Design review of the part shown in the three views and the two pictorial views. Dimensions are in mm from the part's minimum x, y and z. Give positions to 0.01 mm unless a question says otherwise; leave off trailing zeros. Loops run counter-clockwise (first coordinate to the right, second up) from the corner with the lowest first, then second, coordinate; pieces in that order, holes last. Notation, with made-up numbers: (-27, 12.5) - (17, 12.5) arc R17 ccw to (17, 31.5) - close; hole circle Ø6 at (24, 64). An arc over 180 degrees is marked (long way). Answer in a Markdown table with one row per item.
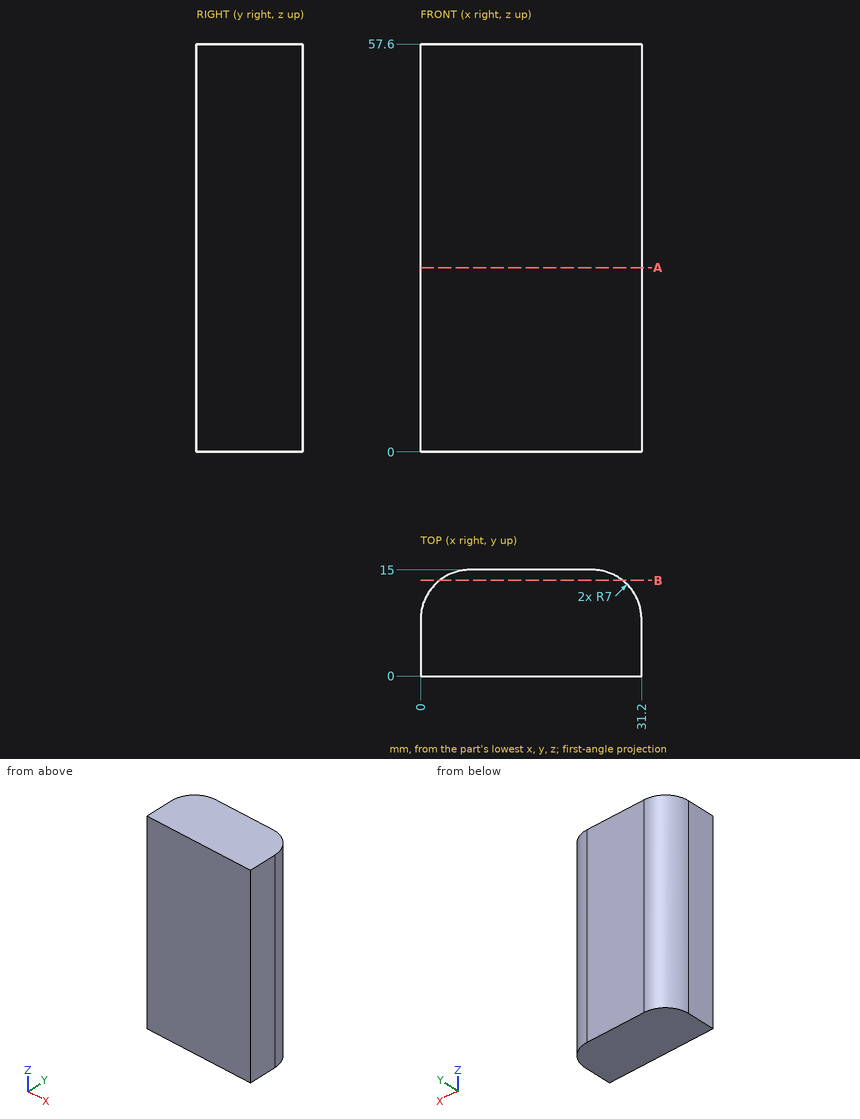
1. Wall thickness on line 1 (Y direction, x = 2, z = 21.5); line 2 (Y direction, x = 27.5, z = 33); line 3 (X direction, y = 11.5, z = 43): over which ranges is each line inside the solid? List them lowest first. Write a range as [from, to].
Values:
| item | result |
|---|---|
| line 1 | y = [0, 12.9] |
| line 2 | y = [0, 14.17] |
| line 3 | x = [0.94, 30.26] |
2. We need section A-A, the plane z = 26. Give the boundary of the cut face in (x, y).
Values:
| item | result |
|---|---|
| outline | (0, 0) - (31.2, 0) - (31.2, 8) arc R7 ccw to (24.2, 15) - (7, 15) arc R7 ccw to (0, 8) - close |
3. We need section B-B, the plane y = 13.5. Give the boundary of the cut face in (x, z).
Values:
| item | result |
|---|---|
| outline | (2.67, 0) - (28.53, 0) - (28.53, 57.6) - (2.67, 57.6) - close |
